```python
from build123d import *

# Parameters (mm, degrees)
CUT_EXTRUDE1_REACH                  = 84.856
CUT_EXTRUDE1_END_RADIUS             = 5
SKETCH3_R                           = 3
CUT_EXTRUDE1_DIRECTION_2_REACH      = 84.856
CUT_EXTRUDE1_DIRECTION_2_END_RADIUS = 5


with BuildPart() as part:
    # Sketch1 → Revolve2 (revolve)
    with BuildSketch(Plane.XY, mode=Mode.PRIVATE) as revolve2_sk:
        Polygon((0, 0), (0, 80), (15.25, 80), (15.25, 76), (13.75, 76), (13.75, 72.5), (15.25, 72.5), (15.25, 68.5), (5, 68.5), (5, 0), align=None)
    revolve(revolve2_sk.sketch.rotate(Axis((0, 0, 0), (0, 1, 0)), 90), axis=Axis((0, 0, 0), (0, 1, 0)))

    # Cut-Extrude1: up to this cylinder (the profile starts inside it)
    cut_extrude1_end = Plane(origin=(0, 10, 0), z_dir=(0, -1, 0)) * Cylinder(CUT_EXTRUDE1_END_RADIUS, 180.712, mode=Mode.PRIVATE)
    # Sketch3 → Cut-Extrude1 (cut, up to the surface)
    with BuildSketch(Plane.XY, mode=Mode.PRIVATE) as cut_extrude1_sk1:
        with Locations(Location((0, 10, 0), (0, 0, 180))):
            Circle(SKETCH3_R)
    cut_extrude1_tool1 = extrude(cut_extrude1_sk1.sketch, amount=-CUT_EXTRUDE1_REACH, mode=Mode.PRIVATE) & cut_extrude1_end
    add(cut_extrude1_tool1.solids().sort_by_distance((0, 10, 0))[0], mode=Mode.SUBTRACT)

    # Cut-Extrude1 direction 2: up to this cylinder (the profile starts inside it)
    cut_extrude1_direction_2_end = Plane(origin=(0, 10, 0), z_dir=(0, -1, 0)) * Cylinder(CUT_EXTRUDE1_DIRECTION_2_END_RADIUS, 180.712, mode=Mode.PRIVATE)
    # Sketch3 → Cut-Extrude1 direction 2 (cut, up to the surface)
    with BuildSketch(Plane.XY, mode=Mode.PRIVATE) as cut_extrude1_direction_2_sk1:
        with Locations(Location((0, 10, 0), (0, 0, 180))):
            Circle(SKETCH3_R)
    cut_extrude1_direction_2_tool1 = extrude(cut_extrude1_direction_2_sk1.sketch, amount=CUT_EXTRUDE1_DIRECTION_2_REACH, mode=Mode.PRIVATE) & cut_extrude1_direction_2_end
    add(cut_extrude1_direction_2_tool1.solids().sort_by_distance((0, 10, 0))[0], mode=Mode.SUBTRACT)


solid = part.part
```
Geometry check sheet. Reference: the model listing, model coordinates, mm. A direction names the side the tool comes from. Coordinates: 2 decimals unless noted, no trailing zeros. Order: outer loops, then holes, each group sorted by start corner. A loop starts at its lowest first (then second) coordinate and runs counter-clockwise, first axis right, second up. Notation, with made-up numbers: (87, 73.25) - (141, 73.25) arc R25 cw to (141, 107.25) - close; hole circle Ø9 at (25, 45). An arc over 180 degrees is marked (long way). Answer in a Markdown table with one row per item. Add a question column.
1. Section check B-B (x = 0). Enter the section's corners in (y, z), plus the area to 3 significant figures.
2. Section check D-D (x = -8.5). Enter the section's corners in (y, z).
3. Section check C-C (y = 10). Enter the section's corners in (x, z), plus the area to 3 significant figures.
4. Access from +Z, -Z, +X, -X, +Y, -Y to the whole of each face (thin tool, end or side, straight path). Record for faces 4 (the face through (14.887, 77.972, 3.306)), 5 (the face through (-4, 68.5, 4)), 6 (the face through (-14, 72.5, -2)).
5. Gauge pin test, flat ends, axial feed: pin 1 Ø8 at (x, y) = (5, 68) entering from +Z; pin 2 Ø7 at (x, y) = (0, 10) entering from +Z; pin 3 Ø1.5 at (x, y) = (3, 56.5) entering from +Z. Record the tip position at first contact, or that the pin passes through.
6. Section check A-A (z = 0). Enter the section's corners in (x, y).
7. Material ranges on L1, parallel to Y at x = 0, z = -0.5; L2, parallel to Y at x = -10, z = -10.5; L3, parallel to Z at x = 4, y = 8, recorded low to high. Write a range as [from, to].
8. Draft check along X on faces 1 (the face through (3, 10, 0)), 2 (the face through (-14, 76, 2)), 3 (the face through (0, 34, 5)). Enter one of: +X half, -X half, draft (parallel to the pull), parting line (faces both ways), or undercut.
Data:
| question | item | result |
|---|---|---|
| 1 | outline | (0, -5) - (7, -5) - (7, 5) - (0, 5) - close; (13, -5) - (68.5, -5) - (68.5, -15.25) - (72.5, -15.25) - (72.5, -13.75) - (76, -13.75) - (76, -15.25) - (80, -15.25) - (80, 15.25) - (76, 15.25) - (76, 13.75) - (72.5, 13.75) - (72.5, 15.25) - (68.5, 15.25) - (68.5, 5) - (13, 5) - close |
| 1 | area | 965 mm² |
| 2 | outline | (68.5, -12.66) - (72.5, -12.66) - (72.5, -10.81) - (76, -10.81) - (76, -12.66) - (80, -12.66) - (80, 12.66) - (76, 12.66) - (76, 10.81) - (72.5, 10.81) - (72.5, 12.66) - (68.5, 12.66) - close |
| 3 | outline | (-3, -4) - (-3, 4) arc R5 ccw to start; (3, -4) arc R5 ccw to (3, 4) - close |
| 3 | area | 22.4 mm² |
| 4 | face 4 | +Y, -Y |
| 4 | face 5 | -Y |
| 4 | face 6 | none |
| 5 | pin 1 | stops at z = 15.22 |
| 5 | pin 2 | stops at z = 5 |
| 5 | pin 3 | stops at z = 4.47 |
| 6 | outline | (-15.25, 68.5) - (-5, 68.5) - (-5, 0) - (5, 0) - (5, 68.5) - (15.25, 68.5) - (15.25, 72.5) - (13.75, 72.5) - (13.75, 76) - (15.25, 76) - (15.25, 80) - (-15.25, 80) - (-15.25, 76) - (-13.75, 76) - (-13.75, 72.5) - (-15.25, 72.5) - close; hole circle Ø6 at (0, 10) |
| 7 | L1 | y = [0, 7], [13, 80] |
| 7 | L2 | y = [68.5, 72.5], [76, 80] |
| 7 | L3 | z = [-3, 3] |
| 8 | face 1 | undercut |
| 8 | face 2 | draft |
| 8 | face 3 | parting line |
